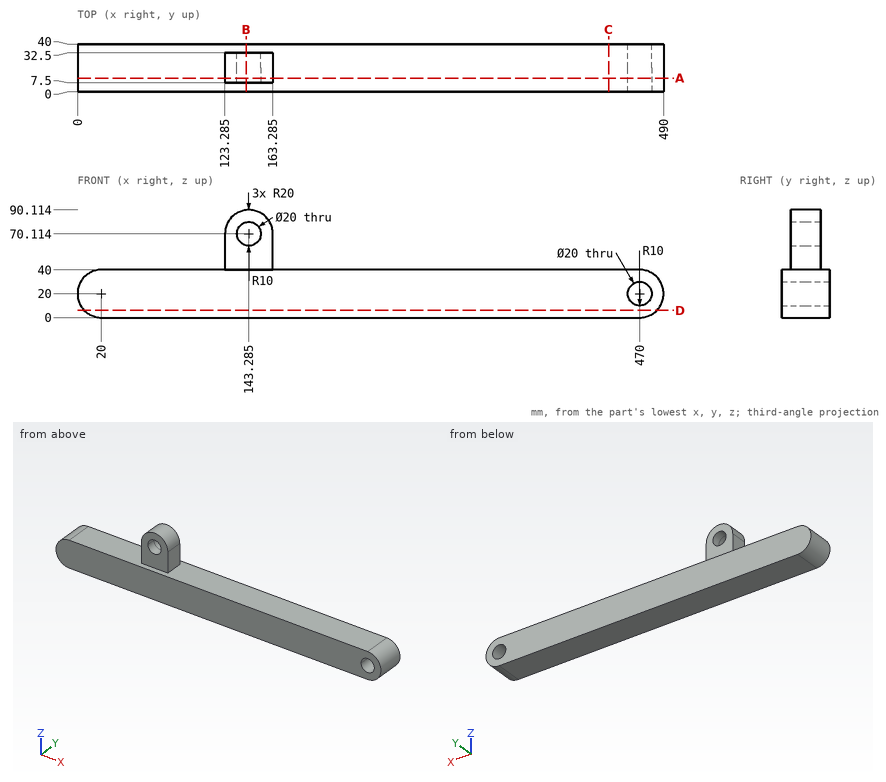
Verification items for this drawing (mm, ordinates from the low corner). Coordinates: 2 decimals unless noted, no trailing zeros. Order: outer loops, then holes, each group sorted by start corner. A loop starts at its lowest first (then second) coordinate and runs counter-clockwise, first axis right, second up. Notation, with made-up numbers: (-29.75, -22) -> (25.25, -22) arc R18 cw to (25.25, -2) -> close; hole circle Ø7 at (50.5, -8.75). An arc over 180 degrees is marked (long way). Put each result on its own line as item: value. Start each with the question number.
1. Go/stop test with flat-tipped pins: pin 1 Ø1 at (y, z) = (10.5, 36) entering from +X; pin 2 Ø5 at (x, y) = (208.5, 14.5) entering from +Z; pin 3 Ø6 at (y, z) = (8, 50) entering from -X (3 decimals). Record where each tip stops, or that it passes through.
2. Cross-section at D-D, the plane z = 6. Record the boundary of the cut face in (x, y).
3. Cross-section at A-A, the plane y = 11.5. Record the boundary of the cut face in (x, z) (3 decimals), then the cut area to 3 significant figures.
4. Cross-section at B-B, the plane x = 141. Record the boundary of the cut face in (y, z), then the cut area to 3 significant figures.
5. Material ranges on L1, parallel to Z at x = 470, y = 29; L2, parallel to X at y = 28, z = 20; L3, parallel to Z at x = 256.5, y = 12.5, recorded low to high. Write a range as [from, to].
6. Cross-section at C-C, the plane x = 444. Record the boundary of the cut face in (y, z).
Computed:
1. pin 1: x = 482.64
1. pin 2: z = 40
1. pin 3: x = 123.285
2. outline: (5.72, 0) -> (484.28, 0) -> (484.28, 40) -> (5.72, 40) -> close
3. outline: (20, 0) -> (470, 0) arc R20 ccw to (470, 40) -> (163.285, 40) -> (163.285, 70.114) arc R20 ccw to (123.285, 70.114) -> (123.285, 40) -> (20, 40) arc R20 ccw to start; hole circle Ø20 at (143.285, 70.114); hole circle Ø20 at (470, 20)
3. area: 20,500 mm2
4. outline: (0, 0) -> (40, 0) -> (40, 40) -> (32.5, 40) -> (32.5, 60.38) -> (7.5, 60.38) -> (7.5, 40) -> (0, 40) -> close; (7.5, 79.85) -> (32.5, 79.85) -> (32.5, 89.98) -> (7.5, 89.98) -> close
4. area: 2,360 mm2
5. L1: [0, 10], [30, 40]
5. L2: [0, 460], [480, 490]
5. L3: [0, 40]
6. outline: (0, 0) -> (40, 0) -> (40, 40) -> (0, 40) -> close
